Read the model definition and answer for the solid it produces. Units are mm, in the model's axes. A direction names the side the tool comes from. Round coordinates to 2 decimals unless told otherwise and drop trailing zeros. Order: outer loops, then holes, each group sorted by start corner. A loop starts at its lowest first (then second) coordinate and runs counter-clockwise, first axis right, second up. Notation, with made-up numbers: (71.25, -34.75) -> (92.25, -34.75) arc R18 ccw to (92.25, -15.75) -> close; hole circle Ø3 at (-5, 54.5). An arc over 180 degrees is marked (long way). Answer as a JSON object with one key per item and string values. Group by question number.
Item 1: Section B-B, the plane x = 19 is taken. Write down the section's boundary in (y, z), plus the area to 3 significant figures.
Item 2: Consider probe 1 along Z at (x, y) = (102.5, 6.75); probe 2 along Z at (x, y) = (43, -1); probe 3 along Y at (x, z) = (49, 11.25). Determine where each line is inside the solid, lowest interval first. Write a range as from..to.
Item 3: Given P1, Ø2, axis at x = 8.5, y = -0.5, coming from the +Z side; P2, Ø1, axis at x = 79, y = -1.5, coming from the +Z side; P3, Ø1, axis at x = 79, y = -1, coming from the -Z side; P4, Ø0.6, axis at y = -1.5, z = 10.5, coming from the -X side, each flat-ended and moving along its own axis, determine where each tip first touches the part or whether it passes through.
Item 4: Section C-C, the plane x = 72 is taken. Write down the section's boundary in (y, z), plus the area to 3 significant figures.
Item 5: The mould has two halves that part along X. Classify faces 4 (the flat face through (8, -1, 4)), 5 (the flat face through (62.6, 0, 0.8)): pulls with the +X half, pulls with the -X half, needs draft (parallel to the pull), parting line crosses it, or undercut.
Item 6: Section A-A, the plane y = 10 is taken. Count the separate pieces of the cut face and the enclosed holes in it, plus the area to 3 significant figures.
Item 7: For faces 1 (the flat face through (40, 9, 7)), 2 (the flat face through (55, 7, 15)), 3 (the flat face through (79, -1, 9.5)), determine the directions among +Z, -Z, +X, -X, +Y, -Y from which every point of the face is accessible in a straight line to the end or side of a thin tool.
from build123d import *

# Parameters (mm, degrees)
SKETCH1_W                   = 8
SKETCH1_H                   = 15
FIRST_CHAMBER_BLOCK_DEPTH   = 15
SKETCH2_W                   = 6
SKETCH2_H                   = 11
FIRST_CHAMBER_CAVITY_DEPTH  = 13
SKETCH3_W                   = 15
SKETCH3_H                   = 3
CHAMBER_SPACER_DEPTH        = 2
PATTERN_CHAMBERS_COUNT      = 11
PATTERN_CHAMBERS_PITCH      = 10
SKETCH4_W                   = 15
SKETCH4_H                   = 12
THICKEN_END_1_DEPTH         = 2
SKETCH5_W                   = 15
SKETCH5_H                   = 15
THICKEN_END_2_DEPTH         = 2
SKETCH6_W                   = 94
SKETCH6_H                   = 2
CENTRAL_AIR_CHANNEL_DEPTH   = 2
SKETCH7_W                   = 108
SKETCH7_H                   = 13
SKETCH7_W_2                 = 106
SKETCH7_H_2                 = 11
BONDING_RIDGE_DEPTH         = 2
SKETCH9_W                   = 2
SKETCH9_H                   = 2.5
BONDING_BUMPS_DEPTH         = 2
PATTERN_BONDING_BUMPS_COUNT = 10
PATTERN_BONDING_BUMPS_PITCH = 10


with BuildPart() as part:
    # Sketch1 → first chamber block (new body)
    with BuildSketch(Plane.XY):
        with Locations((4, 7.5)):
            Rectangle(SKETCH1_W, SKETCH1_H)
    extrude(amount=FIRST_CHAMBER_BLOCK_DEPTH)

    # Sketch2 → first chamber cavity (cut)
    with BuildSketch(Plane.XZ):
        with Locations((4, 7.5)):
            Rectangle(SKETCH2_W, SKETCH2_H)
    extrude(amount=-FIRST_CHAMBER_CAVITY_DEPTH, mode=Mode.SUBTRACT)

    # Sketch3 → chamber spacer (add)
    with BuildSketch(Plane(origin=(8, 0, 0), x_dir=(0, 0, -1), z_dir=(1, 0, 0))):
        with Locations((-7.5, 1.5)):
            Rectangle(SKETCH3_W, SKETCH3_H)
    extrude(amount=CHAMBER_SPACER_DEPTH)


with BuildPart() as pattern_chambers_1:
    # pattern chambers: pattern copy
    add(part.part.moved(Location(Vector(1, 0, 0) * (1 * PATTERN_CHAMBERS_PITCH))))


with BuildPart() as pattern_chambers_2:
    # pattern chambers: pattern copy
    add(part.part.moved(Location(Vector(1, 0, 0) * (2 * PATTERN_CHAMBERS_PITCH))))


with BuildPart() as pattern_chambers_3:
    # pattern chambers: pattern copy
    add(part.part.moved(Location(Vector(1, 0, 0) * (3 * PATTERN_CHAMBERS_PITCH))))


with BuildPart() as pattern_chambers_4:
    # pattern chambers: pattern copy
    add(part.part.moved(Location(Vector(1, 0, 0) * (4 * PATTERN_CHAMBERS_PITCH))))


with BuildPart() as pattern_chambers_5:
    # pattern chambers: pattern copy
    add(part.part.moved(Location(Vector(1, 0, 0) * (5 * PATTERN_CHAMBERS_PITCH))))


with BuildPart() as pattern_chambers_6:
    # pattern chambers: pattern copy
    add(part.part.moved(Location(Vector(1, 0, 0) * (6 * PATTERN_CHAMBERS_PITCH))))


with BuildPart() as pattern_chambers_7:
    # pattern chambers: pattern copy
    add(part.part.moved(Location(Vector(1, 0, 0) * (7 * PATTERN_CHAMBERS_PITCH))))


with BuildPart() as pattern_chambers_8:
    # pattern chambers: pattern copy
    add(part.part.moved(Location(Vector(1, 0, 0) * (8 * PATTERN_CHAMBERS_PITCH))))


with BuildPart() as pattern_chambers_9:
    # pattern chambers: pattern copy
    add(part.part.moved(Location(Vector(1, 0, 0) * (9 * PATTERN_CHAMBERS_PITCH))))


with BuildPart() as pattern_chambers_10:
    # pattern chambers: pattern copy
    add(part.part.moved(Location(Vector(1, 0, 0) * (10 * PATTERN_CHAMBERS_PITCH))))

    # combine into 1 solid body: union pattern chambers_9, pattern chambers_8, pattern chambers_7, pattern chambers_6, pattern chambers_5, pattern chambers_4, pattern chambers_3, pattern chambers_2, pattern chambers_1, part
    add(pattern_chambers_9.part)
    add(pattern_chambers_8.part)
    add(pattern_chambers_7.part)
    add(pattern_chambers_6.part)
    add(pattern_chambers_5.part)
    add(pattern_chambers_4.part)
    add(pattern_chambers_3.part)
    add(pattern_chambers_2.part)
    add(pattern_chambers_1.part)
    add(part.part)

    # Sketch4 → thicken end 1 (add)
    with BuildSketch(Plane(origin=(108, 0, 0), x_dir=(0, 0, -1), z_dir=(1, 0, 0))):
        with Locations((-7.5, 9)):
            Rectangle(SKETCH4_W, SKETCH4_H)
    extrude(amount=THICKEN_END_1_DEPTH)

    # Sketch5 → thicken end 2 (add)
    with BuildSketch(Plane.ZY):
        with Locations((7.5, 7.5)):
            Rectangle(SKETCH5_W, SKETCH5_H)
    extrude(amount=THICKEN_END_2_DEPTH)

    # Sketch6 → central air channel (cut)
    with BuildSketch(Plane.XZ):
        with Locations((54, 7.5)):
            Rectangle(SKETCH6_W, SKETCH6_H)
    extrude(amount=-CENTRAL_AIR_CHANNEL_DEPTH, mode=Mode.SUBTRACT)

    # Sketch7 → bonding ridge (add)
    with BuildSketch(Plane.XZ):
        with Locations((54, 7.5)):
            Rectangle(SKETCH7_W, SKETCH7_H)
        with Locations((54, 7.5)):
            Rectangle(SKETCH7_W_2, SKETCH7_H_2, mode=Mode.SUBTRACT)
    extrude(amount=BONDING_RIDGE_DEPTH)

    # Sketch9 → bonding bumps (add)
    with BuildSketch(Plane.XZ):
        with Locations((9, 10.75)):
            Rectangle(SKETCH9_W, SKETCH9_H)
        with Locations((9, 4.25)):
            Rectangle(SKETCH9_W, SKETCH9_H)
    bonding_bumps = extrude(amount=BONDING_BUMPS_DEPTH)

    # pattern bonding bumps: bonding bumps ×10
    with Locations(*[(i * PATTERN_BONDING_BUMPS_PITCH, 0, 0) for i in range(1, PATTERN_BONDING_BUMPS_COUNT)]):
        add(bonding_bumps)


solid = pattern_chambers_10.part
Values found:
{
 "1": {"outline": "(-2, 1) -> (0, 1) -> (0, 0) -> (3, 0) -> (3, 15) -> (0, 15) -> (0, 14) -> (-2, 14) -> (-2, 13) -> (0, 13) -> (0, 12) -> (-2, 12) -> (-2, 9.5) -> (0, 9.5) -> (0, 8.5) -> (2, 8.5) -> (2, 6.5) -> (0, 6.5) -> (0, 5.5) -> (-2, 5.5) -> (-2, 3) -> (0, 3) -> (0, 2) -> (-2, 2) -> close", "area": "55.0 mm2"},
 "2": {"probe 1": "0..2, 13..15", "probe 2": "1..2, 13..14", "probe 3": "-2..3"},
 "3": {"P1": "z = 15", "P2": "z = 14", "P3": "z = 1", "P4": "x = 0"},
 "4": {"outline": "(-2, 1) -> (0, 1) -> (0, 0) -> (15, 0) -> (15, 15) -> (0, 15) -> (0, 14) -> (-2, 14) -> (-2, 13) -> (13, 13) -> (13, 2) -> (-2, 2) -> close", "area": "86.0 mm2"},
 "5": {"face 4": "undercut", "face 5": "needs draft"},
 "6": {"separate pieces": "11", "enclosed holes": "11", "area": "654 mm2"},
 "7": {"face 1": "+Z, -Z, +Y", "face 2": "+Z, +X, -X, +Y, -Y", "face 3": "-Y"}
}
